```python
from build123d import *

# Parameters (mm, degrees)
F0_R     = 23.8125
F1_DEPTH = 3.175
F3_DEPTH = 0.396875
F5_DEPTH = 0.396875


with BuildPart() as f1:
    # F0 (on Top) → F1 (new body)
    with BuildSketch(Plane.XY):
        Circle(F0_R)
    extrude(amount=F1_DEPTH)

    # F2 (on face) → F3 (cut)
    with BuildSketch(Plane.XY.offset(3.175)):
        with BuildLine():
            Line((-12.6909213141, 1.4016369823), (-12.6909213141, 2.2456407605))
            Line((-12.6909213141, 2.2456407605), (-17.5391789526, 2.2456407605))
            add(Edge.make_bspline(
                [(-17.5391789526, 2.2456407605), (-17.6559062181, 2.2476718851), (-17.9354688339, 2.2554253264), (-18.4402822828, 2.2027182518), (-18.8679220579, 2.0222176003), (-19.1434560116, 1.7706610474), (-19.239281151, 1.5597691872), (-19.2786330359, 1.3259163628), (-19.2712876113, 1.2030485875), (-19.2709770054, 1.1491293553)],
                knots=[0, 0, 0, 0, 0.1560804266, 0.3350119598, 0.5061176479, 0.6557447948, 0.7748919756, 0.8954698873, 1, 1, 1, 1], degree=3))
            Line((-19.2709770054, 1.1491293553), (-19.2709770054, -0.3065037017))
            add(Edge.make_bspline(
                [(-17.5391789526, -1.4030151069), (-17.6559062181, -1.4050462315), (-17.9354688339, -1.4127996728), (-18.4402822828, -1.3600925982), (-18.8679220579, -1.1795919467), (-19.1434560116, -0.9280353938), (-19.239281151, -0.7171435336), (-19.2786330359, -0.4832907092), (-19.2712876113, -0.3604229339), (-19.2709770054, -0.3065037017)],
                knots=[0, 0, 0, 0, 0.1560804266, 0.3350119598, 0.5061176479, 0.6557447948, 0.7748919756, 0.8954698873, 1, 1, 1, 1], degree=3))
            Line((-17.5391789526, -1.4030151069), (-12.6909213141, -1.4030151069))
            Line((-12.6909213141, -1.4030151069), (-12.6909213141, -0.5590113287))
            Line((-12.6909213141, -0.5590113287), (-17.5391789526, -0.5590113287))
            ThreePointArc((-17.5391789526, -0.5590113287), (-17.7177288079, -0.4850535571), (-17.7916865796, -0.3065037017))
            Line((-17.7916865796, -0.3065037017), (-17.7916865796, 1.1491293553))
            ThreePointArc((-17.7916865796, 1.1491293553), (-17.7177288079, 1.3276792107), (-17.5391789526, 1.4016369823))
            Line((-17.5391789526, 1.4016369823), (-12.6909213141, 1.4016369823))
        make_face()
    extrude(amount=-F3_DEPTH, mode=Mode.SUBTRACT)

    # F4 (on face) → F5 (cut)
    with BuildSketch(Plane.XY.offset(3.175)):
        with BuildLine():
            add(Edge.make_bspline(
                [(-6.4630292664, 2.2452620324), (-6.333486021, 2.2475161627), (-5.9516659265, 2.2519011177), (-5.480629737, 2.2050980583), (-5.0429762822, 2.0234611453), (-4.7702874415, 1.7724714993), (-4.673882058, 1.5612964459), (-4.6346702869, 1.3280855562), (-4.6419952443, 1.2038344916), (-4.6423006894, 1.1508111508)],
                knots=[0, 0, 0, 0, 0.1732171564, 0.3460610241, 0.5143237171, 0.6614647441, 0.7786322429, 0.8972067004, 1, 1, 1, 1], degree=3))
            Line((-6.4630292664, 2.2452620324), (-10.2095292664, 2.2452620324))
            add(Edge.make_bspline(
                [(-10.2095292664, 2.2452620324), (-10.3390725118, 2.2475161627), (-10.7208926063, 2.2519011177), (-11.1919287958, 2.2050980583), (-11.6295822506, 2.0234611453), (-11.9022710913, 1.7724714993), (-11.9986764749, 1.5612964459), (-12.0378882459, 1.3280855562), (-12.0305632885, 1.2038344916), (-12.0302578434, 1.1508111508)],
                knots=[0, 0, 0, 0, 0.1732171564, 0.3460610241, 0.5143237171, 0.6614647441, 0.7786322429, 0.8972067004, 1, 1, 1, 1], degree=3))
            Line((-12.0302578434, 1.1508111508), (-12.0302578434, -0.3022970803))
            add(Edge.make_bspline(
                [(-10.2095292664, -1.3967479619), (-10.3390725118, -1.3990020922), (-10.7208926063, -1.4033870472), (-11.1919287958, -1.3565839878), (-11.6295822506, -1.1749470748), (-11.9022710913, -0.9239574288), (-11.9986764749, -0.7127823754), (-12.0378882459, -0.4795714857), (-12.0305632885, -0.3553204211), (-12.0302578434, -0.3022970803)],
                knots=[0, 0, 0, 0, 0.1732171564, 0.3460610241, 0.5143237171, 0.6614647441, 0.7786322429, 0.8972067004, 1, 1, 1, 1], degree=3))
            Line((-10.2095292664, -1.3967479619), (-6.4630292664, -1.3967479619))
            add(Edge.make_bspline(
                [(-6.4630292664, -1.3967479619), (-6.333486021, -1.3990020922), (-5.9516659265, -1.4033870472), (-5.480629737, -1.3565839878), (-5.0429762822, -1.1749470748), (-4.7702874415, -0.9239574288), (-4.673882058, -0.7127823754), (-4.6346702869, -0.4795714857), (-4.6419952443, -0.3553204211), (-4.6423006894, -0.3022970803)],
                knots=[0, 0, 0, 0, 0.1732171564, 0.3460610241, 0.5143237171, 0.6614647441, 0.7786322429, 0.8972067004, 1, 1, 1, 1], degree=3))
            Line((-4.6423006894, -0.3022970803), (-4.6423006894, 1.1508111508))
        make_face()
        with BuildLine():
            ThreePointArc((-10.4635292664, 1.2034273241), (-10.3732916273, 1.3519736494), (-10.2095292664, 1.4102036366))
            Line((-10.2095292664, 1.4102036366), (-6.4630292664, 1.4102036366))
            ThreePointArc((-6.4630292664, 1.4102036366), (-6.2994040409, 1.3521173307), (-6.2090292664, 1.2038620324))
            Line((-6.2090292664, 1.2038620324), (-6.2090292664, -0.3553479619))
            ThreePointArc((-6.2090292664, -0.3553479619), (-6.3117594773, -0.47474039), (-6.4628336175, -0.519289826))
            Line((-6.4628336175, -0.519289826), (-10.2095292664, -0.519289826))
            ThreePointArc((-10.2095292664, -0.519289826), (-10.3608035682, -0.4746109766), (-10.4635292664, -0.3549132536))
            Line((-10.4635292664, -0.3549132536), (-10.4635292664, 1.2034273241))
        make_face(mode=Mode.SUBTRACT)
    extrude(amount=-F5_DEPTH, mode=Mode.SUBTRACT)


solid = f1.part
```
Build history of the part. All positions in model axes, mm. A direction names the side the tool comes from. Round coordinates to 2 decimals unless told otherwise and drop trailing zeros. Order: outer loops, then holes, each group sorted by start corner. A loop starts at its lowest first (then second) coordinate and runs counter-clockwise, first axis right, second up. Notation, with made-up numbers: (8.25, -30.75) -> (61.25, -30.75) arc R12 cw to (61.25, -23.75) -> close; hole circle Ø4 at (-22, 39.5). An arc over 180 degrees is marked (long way). Answer in a Markdown table with one row per item.
1) Band-saw the part on A-A on z = 1.25. Give the cut face in (x, y) (1 decimal).
Values:
| item | result |
|---|---|
| outline | circle Ø47.6 at (0, 0) |
2) Band-saw the part on C-C on x = 12. Give the cut face in (y, z) (3 decimals).
Values:
| item | result |
|---|---|
| outline | (-20.568, 0) -> (20.568, 0) -> (20.568, 3.175) -> (-20.568, 3.175) -> close |
3) Which spindle directions (+Z, -Z, +X, -X, +Y, -Y) get a long thin tool onto all of the face, cutting with end or side? Do faces 4 (the flat face through (-8, 0, 3.175)), 5 (the flat face through (-17, 2, 2.778)). Say none if no direction does.
Values:
| item | result |
|---|---|
| face 4 | +Z, +X, -X, +Y, -Y |
| face 5 | +Z |
4) Mould opens along Y. For faces 1 (the flat face through (-8, -1, 2.778)), 2 (the flat face through (0, 0, 0)), 3 (the cylindrical face through (-18.897, -14.49, 1.565)) say: released by +Y, released by -Y, zero draft, split by the parting line, or undercut.
Values:
| item | result |
|---|---|
| face 1 | undercut |
| face 2 | zero draft |
| face 3 | split by the parting line |
5) Wall check: L1, parallel to Y at x = 0, z = 2.55; L2, parallel to X at y = -15.5, z = 0.6; L3, parallel to X at y = 4.5, z = 2.95. Give the ranges that are in metal, low to high.
Values:
| item | result |
|---|---|
| L1 | -23.81 to 23.81 |
| L2 | -18.08 to 18.08 |
| L3 | -23.38 to 23.38 |
6) Band-saw the part on B-B on y = -21. Give the cut face in (x, z) (3 decimals), and give its area (3 significant figures).
Values:
| item | result |
|---|---|
| outline | (-11.227, 0) -> (11.227, 0) -> (11.227, 3.175) -> (-11.227, 3.175) -> close |
| area | 71.3 mm2 |
